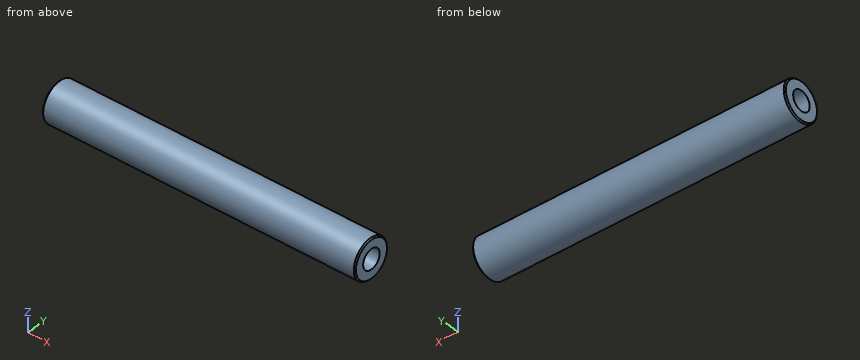
```python
from build123d import *

# Parameters (mm, degrees)
SKETCH_1_W             = 80
SKETCH_1_H             = 5
HOLE_WIZARD_M6_1_D     = 5
HOLE_WIZARD_M6_1_DEPTH = 15
HOLE_WIZARD_M6_1_TIP   = 1.502151548
HOLE_WIZARD_M6_2_D     = 5
HOLE_WIZARD_M6_2_DEPTH = 15
HOLE_WIZARD_M6_2_TIP   = 1.502151548
CHAMFER_1_SIZE         = 0.3


with BuildPart() as part:
    # 草图1 → 旋转1 (revolve)
    with BuildSketch(Plane(origin=(0, 0, 0), x_dir=(1, 0, 0), z_dir=(0, 1, 0)), mode=Mode.PRIVATE) as revolve_1_sk:
        with Locations((40, 2.5)):
            Rectangle(SKETCH_1_W, SKETCH_1_H)
    revolve(revolve_1_sk.sketch.rotate(Axis((-1000, 0, 0), (1, 0, 0)), 180), axis=Axis((-1000, 0, 0), (1, 0, 0)))

    # M6 螺纹孔1
    with Locations(Plane(origin=(80, 0, 0), x_dir=(0, 0, -1), z_dir=(1, 0, 0))):
        with Locations((0, 0)):
            Hole(HOLE_WIZARD_M6_1_D / 2, depth=HOLE_WIZARD_M6_1_DEPTH)
            with Locations((0, 0, -(HOLE_WIZARD_M6_1_DEPTH + HOLE_WIZARD_M6_1_TIP / 2))):  # 118° drill point
                Cone(0, HOLE_WIZARD_M6_1_D / 2, HOLE_WIZARD_M6_1_TIP, mode=Mode.SUBTRACT)

    # M6 螺纹孔2
    with Locations(Plane.ZY):
        with Locations((0, 0)):
            Hole(HOLE_WIZARD_M6_2_D / 2, depth=HOLE_WIZARD_M6_2_DEPTH)
            with Locations((0, 0, -(HOLE_WIZARD_M6_2_DEPTH + HOLE_WIZARD_M6_2_TIP / 2))):  # 118° drill point
                Cone(0, HOLE_WIZARD_M6_2_D / 2, HOLE_WIZARD_M6_2_TIP, mode=Mode.SUBTRACT)

    # 倒角1
    chamfer_1_edges = [part.edges().sort_by_distance(p)[0] for p in [
        (80, 0, -5),
        (0, 0, -5),
    ]]
    chamfer(chamfer_1_edges, length=CHAMFER_1_SIZE)


solid = part.part
```
Check sheet for the modelled part. Datum: model origin and axes. Units: mm. Coordinates: 2 decimals unless noted, no trailing zeros. Order: outer loops, then holes, each group sorted by start corner. A loop starts at its lowest first (then second) coordinate and runs counter-clockwise, first axis right, second up. Notation, with made-up numbers: (79.25, 47.5) -> (83.25, 47.5) arc R14 cw to (83.25, 62.5) -> close; hole circle Ø4 at (28.5, 52). An arc over 180 degrees is marked (long way). Write item = value, one per line. Start each with the question number.
1) Cross-section at A-A (x = 75). Enter the section's corners in (y, z).
2) Cross-section at B-B (x = 26.5). Enter the section's corners in (y, z), then the cut area to 3 significant figures.
3) Go/stop test with flat-tipped pins: P1, Ø3, axis at x = 67, y = -2, coming from the -Z side; P2, Ø3, axis at x = 11, y = 3, coming from the -Z side; P3, Ø1, axis at x = 36.5, z = 2, coming from the +Y side. Record where each tip stops, or that it passes through.
4) Material ranges on L1, parallel to Y at x = 76, z = 0; L2, parallel to Y at x = 27, z = -0.25; L3, parallel to Z at x = 34, y = -3.5, recorded low to high.
Ans:
q1.outline = circle Ø10 at (0, 0); hole circle Ø5 at (0, 0)
q2.outline = circle Ø10 at (0, 0)
q2.area = 78.5 mm²
q3.P1 = -4.97
q3.P2 = -4.77
q3.P3 = 4.77
q4.L1 = -5 to -2.5, 2.5 to 5
q4.L2 = -4.99 to 4.99
q4.L3 = -3.57 to 3.57
